Here's how the part is built. I have some questions about the finished solid (model axes, mm). Face numbers are marked on the shaded views. A direction names the side the tool comes from. Coordinates: 2 decimals unless noted, no trailing zeros. Loops run counter-clockwise (first coordinate to the right, second up) from the corner with the lowest first, then second, coordinate; pieces in that order, holes last. Notation, with made-up numbers: (32.25, -38.75) -> (73.25, -38.75) arc R23 ccw to (73.25, -3.75) -> close; hole circle Ø7 at (86, -27). An arc over 180 degrees is marked (long way). Answer as a JSON object with one key per item and string values. Group by question number.
Q1. On a 3-axis mill with a long thin cutter (end or side, diameter ignored), from which of +Z, -Z, +X, -X, +Y, -Y can I reach the whole of each face in a straight line? I mean the marked faces 1 and 2. Say none if no direction works.
Q2. I'm going to push flat-ended pins straight in: pin 1 (1.5 mm diameter, centred on y = 28, z = -21, fed in from -X); pin 2 (1.5 mm diameter, centred on x = -13, y = 6, fed in from +Z); pin 3 (3 mm diameter, centred on x = -25, z = 0, fed in from +Y); pin 4 (10 mm diameter, centred on y = 20, z = 19, fed in from -X). Where does each tip first touch, or does it pass through?
Q3. I want a section at A-A on y = 23. Write out the boundary of the cut face in (x, z), then the cut area to 3 significant figures.
Q4. I want a section at B-B on x = -16.5. Write out the boundary of the cut face in (y, z), then the cut area to 3 significant figures.
Q5. Thinking about a two-plate mould opening in X: for the marked faces 3, 4, 5 and 6, which applies, released by +X, released by -X, zero draft, split by the parting line, or undercut?
Q6. I want a section at C-C on x = 20. Write out the boundary of the cut face in (y, z), then the cut area to 3 significant figures.
Q7. I want a section at D-D on y = 13.5. Write out the boundary of the cut face in (x, z).
Q8. I need wall thicknesses on line 1 (X direction, y = 31, z = 0); line 2 (X direction, y = 3, z = -13). Which ranges of each line are inside material? Lowest first, please.
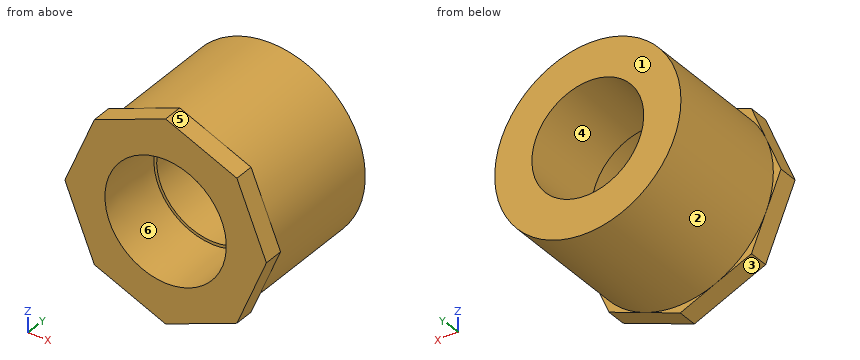
```python
from build123d import *

# Parameters (mm, degrees)
SKETCH1_W           = 17.78
SKETCH1_H           = 38.1
SKETCH2_R           = 6.35
BOSS_EXTRUDE1_DEPTH = 5.0546


with BuildPart() as part:
    # Sketch1 → Revolve1 (revolve)
    with BuildSketch(Plane.XY):
        with Locations((-15.24, 19.05)):
            Rectangle(SKETCH1_W, SKETCH1_H)
    revolve(axis=Axis((0, 0, 0), (0, -1, 0)))

    # Sketch2 → Boss-Extrude1 (add)
    with BuildSketch(Plane.XZ):
        Polygon((0, 26.118123793), (-18.468302446, 18.468302446), (-26.118123793, 0), (-18.468302446, -18.468302446), (0, -26.118123793), (18.468302446, -18.468302446), (26.118123793, 0), (18.468302446, 18.468302446), align=None)
        Circle(SKETCH2_R, mode=Mode.SUBTRACT)
    extrude(amount=-BOSS_EXTRUDE1_DEPTH)

    # Sketch4 → 1 NPT Tapped Hole1 (revolve, cut)
    with BuildSketch(Plane(origin=(0, 0, 0), x_dir=(0, 0, -1), z_dir=(1, 0, 0))):
        Polygon((0, 0), (0, 38.1), (14.4907, 38.1), (14.4907, 16.78686), (15.227979931, 16.78686), (15.730601, 0), align=None)
    revolve(axis=Axis((0, -6.35, 0), (0, 1, 0)), mode=Mode.SUBTRACT)


solid = part.part
```
Result set:
{
 "1": {"face 1": "+Z, -Z, +X, -X, +Y", "face 2": "+Y"},
 "2": {"pin 1": "stops at x = -13.12", "pin 2": "stops at z = 20.79", "pin 3": "stops at y = 38.1", "pin 4": "stops at x = -19.65"},
 "3": {"outline": "circle Ø48.26 at (0, 0); hole circle Ø28.98 at (0, 0)", "area": "1,170 mm²"},
 "4": {"outline": "(0, -19.28) -> (5.05, -19.28) -> (5.05, -17.61) -> (38.1, -17.61) -> (38.1, 17.61) -> (5.05, 17.61) -> (5.05, 19.28) -> (0, 19.28) -> close", "area": "1,360 mm²"},
 "5": {"face 3": "released by -X", "face 4": "undercut", "face 5": "released by +X", "face 6": "undercut"},
 "6": {"outline": "(0, -14.77) -> (5.05, -14.77) -> (5.05, -13.5) -> (38.1, -13.5) -> (38.1, 13.5) -> (5.05, 13.5) -> (5.05, 14.77) -> (0, 14.77) -> close", "area": "1,040 mm²"},
 "7": {"outline": "circle Ø48.26 at (0, 0); hole circle Ø30.65 at (0, 0)"},
 "8": {"line 1": "x = -24.13 to -14.49, 14.49 to 24.13", "line 2": "x = -20.73 to -8.7, 8.7 to 20.73"}
}
